Geometry: see drawing. Coordinates: mm, zero at the bounding-box minimum. A direction names the side the tool comes from. Round coordinates to 2 decimals unless told otherwise and drop trailing zeros. Loops run counter-clockwise (first coordinate to the right, second up) from the corner with the lowest first, then second, coordinate; pieces in that order, holes last. Notation, with made-up numbers: (67.25, -36) -> (111.25, -36) arc R24 ccw to (111.25, -11) -> close; hole circle Ø5 at (-6.75, -29). An arc over 180 degrees is marked (long way). Answer in a Markdown table with one row per item.
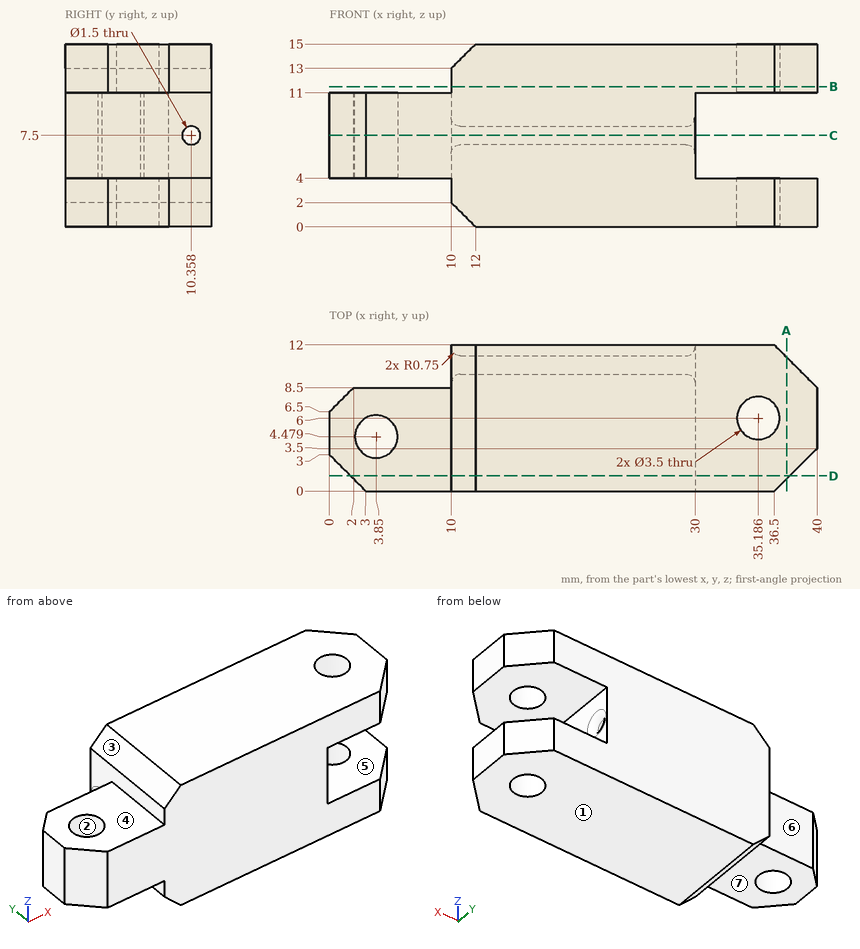
Item 1: First-contact query: P1, Ø5.5, axis at y = 5, z = 7, coming from the +X side; P2, Ø7, axis at x = 5, y = 3, coming from the -Z side; P3, Ø3, axis at x = 35.19, y = 6, coming from the +Z side. Flat tips, straight axial feed; report the tip coordinate or a pass-through.
Ans:
| item | result |
|---|---|
| P1 | x = 30 |
| P2 | z = 4 |
| P3 | through |
Item 2: Section query D-D, the plane y = 1.25. Output: boundary loops of the cut face in (x, z).
Ans:
| item | result |
|---|---|
| outline | (1.75, 4) -> (10, 4) -> (10, 2) -> (12, 0) -> (37.75, 0) -> (37.75, 4) -> (30, 4) -> (30, 11) -> (37.75, 11) -> (37.75, 15) -> (12, 15) -> (10, 13) -> (10, 11) -> (1.75, 11) -> close |
Item 3: Mould query, pull axis X, two halves, no side actions, for the marked faces 1, 2 and 3. Classes: released by +X, released by -X, zero draft, split by the parting line, or undercut.
Ans:
| item | result |
|---|---|
| face 1 | zero draft |
| face 2 | undercut |
| face 3 | released by -X |
Item 4: Ray query, L1, parallel to Z at x = 38.5, y = 3.25; L2, parallel to Y at x = 16, z = 7.5; L3, parallel to Z at x = 9, y = 5.25. Return the intervals inside material, ascending.
Ans:
| item | result |
|---|---|
| L1 | 0 to 4, 11 to 15 |
| L2 | 0 to 9.61, 11.11 to 12 |
| L3 | 4 to 11 |
Item 5: Set-up query: the marked faces 4, 5, 6 and 7. Return all of +Z, -Z, +X, -X, +Y, -Y with unobstructed straight access to the full face (end or side cutting, diameter ignored); none if empty.
Ans:
| item | result |
|---|---|
| face 4 | +Z, -X, +Y, -Y |
| face 5 | +X, +Y, -Y |
| face 6 | +Z, -Z, -X, +Y |
| face 7 | -Z, -X, +Y, -Y |
Item 6: Section query A-A, the plane x = 37.5. Output: boundary loops of the cut face in (y, z).
Ans:
| item | result |
|---|---|
| outline | (1, 0) -> (11, 0) -> (11, 4) -> (1, 4) -> close; (1, 11) -> (11, 11) -> (11, 15) -> (1, 15) -> close |
Item 7: Section query B-B, the plane z = 11.5. Output: boundary loops of the cut face in (x, y).
Ans:
| item | result |
|---|---|
| outline | (10, 0) -> (36.5, 0) -> (40, 3.5) -> (40, 8.5) -> (36.5, 12) -> (10, 12) -> close; hole circle Ø3.5 at (35.19, 6) |
Item 8: Section query C-C, the plane z = 7.5. Output: boundary loops of the cut face in (x, y).
Ans:
| item | result |
|---|---|
| outline | (0, 3) -> (3, 0) -> (30, 0) -> (30, 8.86) arc R0.75 ccw to (29.25, 9.61) -> (10.75, 9.61) arc R0.75 ccw to (10, 8.86) -> (10, 8.5) -> (2, 8.5) -> (0, 6.5) -> close; (10, 11.86) arc R0.75 ccw to (10.75, 11.11) -> (29.25, 11.11) arc R0.75 ccw to (30, 11.86) -> (30, 12) -> (10, 12) -> close; hole circle Ø3.5 at (3.85, 4.48) |
